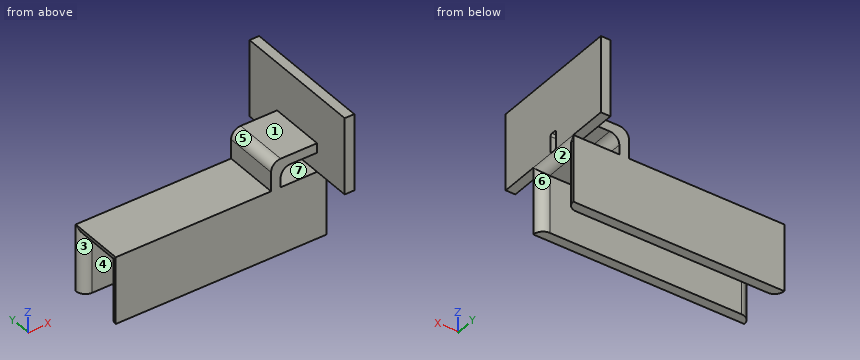
```python
from build123d import *

# Parameters (mm, degrees)
F1_DEPTH = 110
F3_DEPTH = 5
F5_DEPTH = 29
F7_DEPTH = 5
F8_R     = 4.99999
F9_R     = 4.99999


# Not quite as in the source:
# - a fillet or chamfer is up to 0.001 mm smaller than in the source, because OpenCascade refuses the exact size


with BuildPart() as f1:
    # F0 (on Right) → F1 (new body)
    with BuildSketch(Plane.YZ):
        Polygon((-5, -30), (0, -30), (0, 0), (19, 0), (19, -30), (24, -30), (24, 5), (-5, 5), align=None)
    extrude(amount=-F1_DEPTH)

    # F2 (on face) → F3 (join)
    with BuildSketch(Plane.YZ):
        Polygon((-25, 5), (-5, 5), (24, 5), (44, 5), (44, 45), (-25, 45), align=None)
    extrude(amount=-F3_DEPTH)

    # F4 (on face) → F5 (join, through all)
    with BuildSketch(Plane.XZ.offset(5)):
        with BuildLine():
            Line((-19, 15), (-5, 15))
            Line((-5, 15), (-5, 20))
            Line((-5, 20), (-24, 20))
            ThreePointArc((-24, 20), (-27.5355339059, 18.5355339059), (-29, 15))
            Line((-29, 15), (-29, 5))
            Line((-29, 5), (-24, 5))
            Line((-24, 5), (-24, 10))
            ThreePointArc((-24, 10), (-22.5355339059, 13.5355339059), (-19, 15))
        make_face()
    extrude(amount=-F5_DEPTH)

    # F6 (on face) → F7 (cut, through all)
    with BuildSketch(Plane.YZ):
        with BuildLine():
            Line((8.5, 5), (9.5, 5))
            Line((9.5, 5), (10.5, 5))
            ThreePointArc((10.5, 5), (11.2071067812, 5.2928932188), (11.5, 6))
            Line((11.5, 6), (11.5, 14))
            ThreePointArc((11.5, 14), (11.2071067812, 14.7071067812), (10.5, 15))
            Line((10.5, 15), (8.5, 15))
            ThreePointArc((8.5, 15), (7.7928932188, 14.7071067812), (7.5, 14))
            Line((7.5, 14), (7.5, 6))
            ThreePointArc((7.5, 6), (7.7928932188, 5.2928932188), (8.5, 5))
        make_face()
    extrude(amount=-F7_DEPTH, mode=Mode.SUBTRACT)

    # F8 (radius 5 in the source; OpenCascade refuses exactly that, so slightly less here)
    f8_edges = [f1.edges().sort_by_distance(p)[0] for p in [
        (-110, 19, -15),
        (-110, 9.5, 0),
        (-110, 0, -15),
    ]]
    fillet(f8_edges, radius=F8_R)

    # F9 (radius 5 in the source; OpenCascade refuses exactly that, so slightly less here)
    f9_edges = [f1.edges().sort_by_distance(p)[0] for p in [
        (0, 0, -15),
        (0, 19, -15),
        (0, 9.5, 0),
    ]]
    fillet(f9_edges, radius=F9_R)


solid = f1.part
```
Can you work these out from the model? Positions are in its coordinate system, mm. Face numbers are marked on the shaded views. A direction names the side the tool comes from. Coordinates: 2 decimals unless noted, no trailing zeros. Loops run counter-clockwise (first coordinate to the right, second up) from the corner with the lowest first, then second, coordinate; pieces in that order, holes last.
Item 1: Suppose I cut it at A-A (x = -13.5). Please give me the cut outline in (y, z), then the cut area to 3 significant figures.
Answers below:
outline: (-5, -30) - (0, -30) - (0, 0) - (19, 0) - (19, -30) - (24, -30) - (24, 5) - (-5, 5) - close; (-5, 15) - (24, 15) - (24, 20) - (-5, 20) - close
area: 590 mm2
Item 2: Please list where these lines run through material, in increasing order: L1, parallel to Y at x = -90.5, z = -7; L2, parallel to X at y = 5, z = 30; L3, parallel to Z at x = -70.5, y = 0.5.
Answers below:
L1: y = -5 to 0, 19 to 24
L2: x = -5 to 0
L3: z = 0 to 5
Item 3: Suppose I cut it at D-D (z = 39). Please give me the cut outline in (x, y).
Answers below:
outline: (-5, -25) - (0, -25) - (0, 44) - (-5, 44) - close
Item 4: Which directions (+Z, -Z, +X, -X, +Y, -Y) give clear straight access to the entire face, cutting with the end or side of a thin tool? Please do the marked faces 1, 2, 3 and 4.
Answers below:
face 1: +Z, -X, +Y, -Y
face 2: -Z, +X
face 3: -Z, -X
face 4: -Z, +X, -X
Item 5: I'm going to push flat-ended pins straight in: pin 1 (3 mm diameter, centred on y = 2, z = 23.5, fed in from +X); pin 2 (15 mm diameter, centred on x = -15, y = 15, fed in from +Z); pin 3 (15 mm diameter, centred on x = -49.5, z = -5, fed in from +Y); pin 4 (2 mm diameter, centred on x = -52.5, z = -7.5, fed in from -Y). Where does each tip first touch, or does it pass through?
Answers below:
pin 1: stops at x = 0
pin 2: stops at z = 20
pin 3: stops at y = 24
pin 4: stops at y = -5
Item 6: Suppose I cut it at C-C (x = -98). Please give me the cut outline in (y, z).
Answers below:
outline: (-5, -30) - (0, -30) - (0, 0) - (19, 0) - (19, -30) - (24, -30) - (24, 5) - (-5, 5) - close
Item 7: If we mould it in two halves opening along Z, with no side actions, what happens to the marked faces 5, 6 and 7? For each: released by +Z, released by -Z, zero draft, split by the parting line, or undercut.
Answers below:
face 5: released by +Z
face 6: zero draft
face 7: undercut
